Part print with two shaded views. Sizes in mm from the minimum x, y, z corner. A direction names the side the tool comes from. Round coordinates to 2 decimals unless told otherwise and drop trailing zeros. Answer as a JSON object with one key per item and string values. Group by question number.
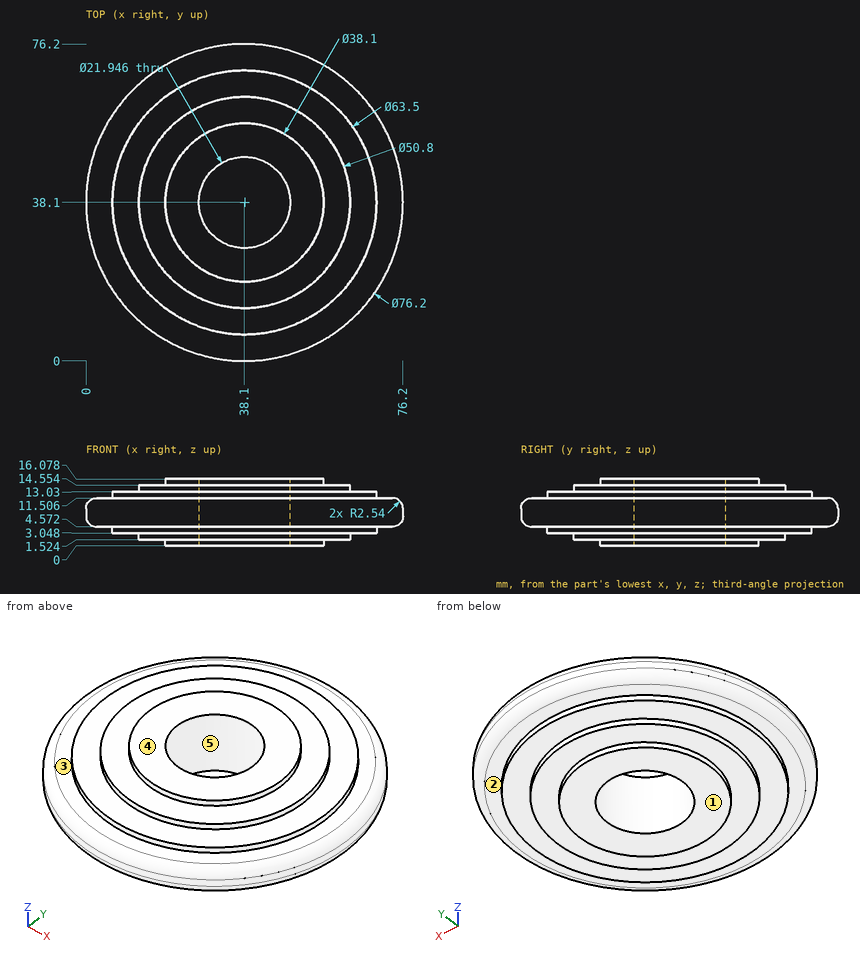
Item 1: Drill centre lines: line 1 (Y direction, x = 38.1, z = 9.25) (1 decimal); line 2 (X direction, y = 38.1, z = 3.75); line 3 (X direction, y = 31.5, z = 12) (1 decimal). Where is each one in solid material? Low to high.
Item 2: Drop flat-ended pins along their axis: pin 1 Ø1.5 at (x, z) = (19.5, 11.5) entering from -Y; pin 2 Ø4 at (y, z) = (43, 9) entering from +X; pin 3 Ø8 at (y, z) = (22.5, 8) entering from +X. Give the stop position or say it passes through.
Item 3: Which spindle directions (+Z, -Z, +X, -X, +Y, -Y) get a long thin tool onto all of the face, cutting with end or side? Do the marked faces 1, 2 and 3. Say none if no direction does.
Item 4: Two-plate mould, pull along X, no slides. Class the marked faces 4 and 5: pulls with the +X half, pulls with the -X half, needs draft (parallel to the pull), parting line crosses it, or undercut.
Entries:
{
 "1": {"line 1": "0 to 27.1, 49.1 to 76.2", "line 2": "6.35 to 27.13, 49.07 to 69.85", "line 3": "7 to 29.3, 46.9 to 69.2"},
 "2": {"pin 1": "y = 5.59", "pin 2": "x = 76.09", "pin 3": "x = 74.39"},
 "3": {"face 1": "-Z, +X, -X, +Y, -Y", "face 2": "-Z", "face 3": "+Z"},
 "4": {"face 4": "needs draft", "face 5": "undercut"}
}
